from build123d import *

# Parameters (mm, degrees)
BOSS_EXTRU_1_DEPTH      = 10
BOSS_EXTRU_2_DEPTH      = 3.8
ESQUISSE3_R             = 1.25
ENL_V_MAT_EXTRU_1_DEPTH = 13


with BuildPart() as part:
    # Esquisse1 → Boss.-Extru.1 (new body)
    with BuildSketch(Plane.XY):
        with BuildLine():
            Line((-12, 0), (0, 0))
            Line((0, 0), (0, 26))
            Line((0, 26), (-12, 26))
            Line((-12, 26), (-12, 21))
            ThreePointArc((-12, 21), (-6.343145751, 18.656854249), (-4, 13))
            ThreePointArc((-4, 13), (-6.343145751, 7.343145751), (-12, 5))
            Line((-12, 5), (-12, 0))
        make_face()
    extrude(amount=BOSS_EXTRU_1_DEPTH)

    # Esquisse2 → Boss.-Extru.2 (add)
    with BuildSketch(Plane.XY.offset(10)):
        with BuildLine():
            ThreePointArc((-12, 5), (-4, 13), (-12, 21))
            Line((-12, 21), (-12, 19))
            ThreePointArc((-12, 19), (-7.757359313, 17.242640687), (-6, 13))
            ThreePointArc((-6, 13), (-7.757359313, 8.757359313), (-12, 7))
            Line((-12, 7), (-12, 5))
        make_face()
    extrude(amount=-BOSS_EXTRU_2_DEPTH)

    # Esquisse3 → Enlèv. mat.-Extru.1 (cut, through all)
    with BuildSketch(Plane.ZY.offset(12)):
        with Locations((3, 23.5)):
            Circle(ESQUISSE3_R)
        with Locations((3, 2.5)):
            Circle(ESQUISSE3_R)
    extrude(amount=-ENL_V_MAT_EXTRU_1_DEPTH, mode=Mode.SUBTRACT)


solid = part.part
Work out the finished part from the listing and answer in its coordinate system (mm). A direction names the side the tool comes from. Round coordinates to 2 decimals unless told otherwise and drop trailing zeros. Order: outer loops, then holes, each group sorted by start corner. A loop starts at its lowest first (then second) coordinate and runs counter-clockwise, first axis right, second up. Notation, with made-up numbers: M -37,35.5 L -1,35.5 A9 ccw -1,43.5 Z; hole C 39,35.5 d7. An arc over 180 degrees is marked long. One line per item, written item: value.
Q1. Find section C-C on x = -7.5. Write down the section's boundary in (y, z), then the cut area to 3 significant figures.
Derived:
outline: M 0,0 L 6.39,0 L 6.39,6.2 L 9.03,6.2 L 9.03,10 L 0,10 Z; M 16.97,6.2 L 19.61,6.2 L 19.61,0 L 26,0 L 26,10 L 16.97,10 Z; hole C 2.5,3 d2.5; hole C 23.5,3 d2.5
area: 138 mm²
Q2. A flat-ended cylindrical pin translates along its axis: pin 1 (6 mm diameter, centred on y = 17.5, z = 4, fed in from -X). Find the tip coordinate at first contact, or state that the pin passes through.
Derived:
pin 1: x = -12
Q3. Find section A-A on z = 3. Write down the section's boundary in (x, y), then the cut area to 3 significant figures.
Derived:
outline: M -12,0 L 0,0 L 0,1.25 L -12,1.25 Z; M -12,3.75 L 0,3.75 L 0,22.25 L -12,22.25 L -12,21 A8 cw -12,5 Z; M -12,24.75 L 0,24.75 L 0,26 L -12,26 Z
area: 151 mm²
Q4. Find section B-B on y = 23.5. Write down the section's boundary in (x, z), then the cut area to 3 significant figures.
Derived:
outline: M -12,0 L 0,0 L 0,1.75 L -12,1.75 Z; M -12,4.25 L 0,4.25 L 0,10 L -12,10 Z
area: 90.0 mm²
Q5. For faces 1 (the face through (-5.6, 12.4, 6.2)), 2 (the face through (0, 13, 5)), determine the directions among +Z, -Z, +X, -X, +Y, -Y from which every point of the face is accessible in a straight line to the end or side of a thin tool.
Derived:
face 1: -Z, -X
face 2: +Z, -Z, +X, +Y, -Y
Q6. Determine the mould class of faces 3 (the face through (-6.08, 22.28, 2.73)), 4 (the face through (-12, 23, 6)), 5 (the face through (-5, 13, 10)) for opening direction Z: released by +Z, released by -Z, zero draft, split by the parting line, or undercut.
Derived:
face 3: undercut
face 4: zero draft
face 5: released by +Z
Q7. Straight lines are drawn through the part: line 1 (Y direction, x = -9, z = 2); line 2 (Y direction, x = -10.5, z = 2.25); line 3 (Z direction, x = -7, y = 3.25). For each, find the intervals that lie inside material, in ascending order.
Derived:
line 1: 0 to 1.75, 3.25 to 5.58, 20.42 to 22.75, 24.25 to 26
line 2: 0 to 1.5, 3.5 to 5.14, 20.86 to 22.5, 24.5 to 26
line 3: 0 to 2, 4 to 10
Q8. Find section D-D on x = -1.25. Write down the section's boundary in (y, z).
Derived:
outline: M 0,0 L 26,0 L 26,10 L 0,10 Z; hole C 2.5,3 d2.5; hole C 23.5,3 d2.5
